Can you work these out from the model? Positions are in its coordinate system, mm. Round coordinates to 2 decimals unless told otherwise and drop trailing zeros. Write each loop counter-clockwise with the first axis right and the second up, starting at its lowest first coordinate (ties: lowest second). Pieces come first, ordered by that corner, then holes. Notation, with made-up numbers: (72, -3) -> (98, -3) arc R19 cw to (98, 2) -> close; hole circle Ø3 at (75, 61). An arc over 180 degrees is marked (long way). Use CSV: the item, a comma, the result in double quotes.
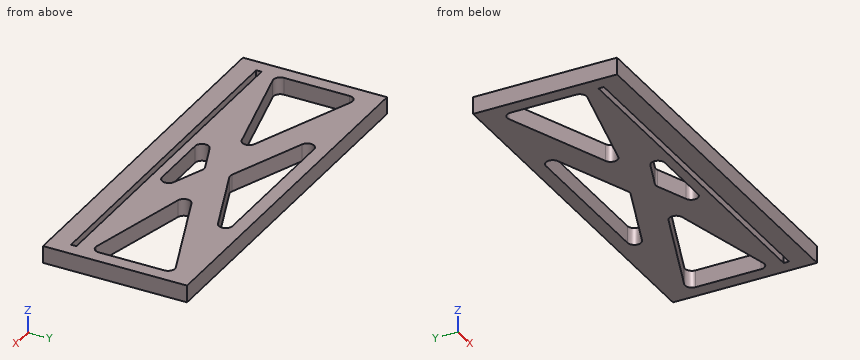
```python
from build123d import *

# Parameters (mm, degrees)
SKETCH1_W           = 68.58
SKETCH1_H           = 26.67
SKETCH1_W_2         = 63.5
SKETCH1_H_2         = 1
BOSS_EXTRUDE1_DEPTH = 3.175
FILLET1_R           = 1.27


with BuildPart() as part:
    # Sketch1 → Boss-Extrude1 (new body)
    with BuildSketch(Plane.XY):
        Rectangle(SKETCH1_W, SKETCH1_H)
        Polygon((-20.750635985, 10.795), (0, 2.725308228), (20.750635985, 10.795), align=None, mode=Mode.SUBTRACT)
        with Locations((0, -9.025)):
            Rectangle(SKETCH1_W_2, SKETCH1_H_2, mode=Mode.SUBTRACT)
        Polygon((-31.75, 9.621913994), (-31.75, -5.985), (-7.007935444, 0), align=None, mode=Mode.SUBTRACT)
        Polygon((7.007935444, 0), (31.75, 9.621913994), (31.75, -5.985), align=None, mode=Mode.SUBTRACT)
        Polygon((0, -1.90771576), (-12.443873761, -6.747), (12.443873761, -6.747), align=None, mode=Mode.SUBTRACT)
    extrude(amount=BOSS_EXTRUDE1_DEPTH)

    # Fillet1
    fillet1_edges = [part.edges().sort_by_distance(p)[0] for p in [
        (20.750635985, 10.795, 1.5875),
        (-20.750635985, 10.795, 1.5875),
        (0, 2.725308228, 1.5875),
        (-7.007935444, 0, 1.5875),
        (-31.75, 9.621913994, 1.5875),
        (-31.75, -5.985, 1.5875),
        (7.007935444, 0, 1.5875),
        (31.75, -5.985, 1.5875),
        (31.75, 9.621913994, 1.5875),
        (12.443873761, -6.747, 1.5875),
        (0, -1.90771576, 1.5875),
        (-12.443873761, -6.747, 1.5875),
    ]]
    fillet(fillet1_edges, radius=FILLET1_R)


solid = part.part
```
Q1. Suppose I cut it at B-B (z = 2.45). Count the separate pieces of the cut face and the enclosed holes in it, and give its area (3 significant figures).
Resolved:
separate pieces,"1"
enclosed holes,"5"
area,"1,190 mm^2"
Q2. Please list where these lines run through material, in increasing order: probe 1 along Y at (x, z) = (-26.5, 1.35) (3 decimals); probe 2 along Y at (x, z) = (-16, 2.55) (3 decimals); probe 3 along Y at (x, z) = (-13.5, 1.55) (3 decimals).
Resolved:
probe 1,"y = -13.335 to -9.525, -8.525 to -4.715, 7.58 to 13.335"
probe 2,"y = -13.335 to -9.525, -8.525 to -2.175, 3.497 to 13.335"
probe 3,"y = -13.335 to -9.525, -8.525 to -1.57, 2.525 to 7.975, 10.795 to 13.335"
Q3. Suppose I cut it at D-D (x = -20). Write out the boundary of the cut face in (y, z) (3 decimals), and give its area (3 significant figures).
Resolved:
outline,"(-13.335, 0) -> (-9.525, 0) -> (-9.525, 3.175) -> (-13.335, 3.175) -> close; (-8.525, 0) -> (-3.143, 0) -> (-3.143, 3.175) -> (-8.525, 3.175) -> close; (5.052, 0) -> (13.335, 0) -> (13.335, 3.175) -> (5.052, 3.175) -> close"
area,"55.5 mm^2"
Q4. Suppose I cut it at A-A (y = 6.5). Write out the boundary of the cut face in (x, z) (3 decimals).
Resolved:
outline,"(-34.29, 0) -> (-31.75, 0) -> (-31.75, 3.175) -> (-34.29, 3.175) -> close; (-23.722, 0) -> (-9.706, 0) -> (-9.706, 3.175) -> (-23.722, 3.175) -> close; (9.706, 0) -> (23.722, 0) -> (23.722, 3.175) -> (9.706, 3.175) -> close; (31.75, 0) -> (34.29, 0) -> (34.29, 3.175) -> (31.75, 3.175) -> close"
Q5. Suppose I cut it at C-C (x = -1.5). Write out the boundary of the cut face in (y, z) (3 decimals), and give its area (3 significant figures).
Resolved:
outline,"(-13.335, 0) -> (-9.525, 0) -> (-9.525, 3.175) -> (-13.335, 3.175) -> close; (-8.525, 0) -> (-6.747, 0) -> (-6.747, 3.175) -> (-8.525, 3.175) -> close; (-2.491, 0) -> (3.309, 0) -> (3.309, 3.175) -> (-2.491, 3.175) -> close; (10.795, 0) -> (13.335, 0) -> (13.335, 3.175) -> (10.795, 3.175) -> close"
area,"44.2 mm^2"
